For this review, take the finished solid that the model builds, in its own axes (mm). Face numbers are marked on the shaded views. A direction names the side the tool comes from. Coordinates: 2 decimals unless noted, no trailing zeros. Write each loop counter-clockwise with the first axis right and the second up, starting at its lowest first coordinate (ties: lowest second). Pieces come first, ordered by that corner, then holes.
```python
from build123d import *

# Parameters (mm, degrees)
SKETCH1_R                       = 6.35
BOSS_EXTRUDE1_DEPTH             = 25.4
F_21_0_159_DIAMETER_HOLE1_D     = 4.0386
F_21_0_159_DIAMETER_HOLE1_DEPTH = 9.0000074
F_21_0_159_DIAMETER_HOLE1_TIP   = 1.213317848
SKETCH5_W                       = 1.35255
SKETCH5_H                       = 6.35
SKETCH7_W                       = 12.7
SKETCH7_H                       = 3.96875


with BuildPart() as part:
    # Sketch1 → Boss-Extrude1 (new body)
    with BuildSketch(Plane(origin=(0, 0, 0), x_dir=(0, 0, -1), z_dir=(1, 0, 0))):
        Circle(SKETCH1_R)
    extrude(amount=BOSS_EXTRUDE1_DEPTH)

    # #21 (0.159) Diameter Hole1
    with Locations(Plane(origin=(25.4, 0, 0), x_dir=(0, 0, -1), z_dir=(1, 0, 0))):
        with Locations((0, 0)):
            Hole(F_21_0_159_DIAMETER_HOLE1_D / 2, depth=F_21_0_159_DIAMETER_HOLE1_DEPTH)
            with Locations((0, 0, -(F_21_0_159_DIAMETER_HOLE1_DEPTH + F_21_0_159_DIAMETER_HOLE1_TIP / 2))):  # 118° drill point
                Cone(0, F_21_0_159_DIAMETER_HOLE1_D / 2, F_21_0_159_DIAMETER_HOLE1_TIP, mode=Mode.SUBTRACT)

    # Sketch5 → #6-32 Tapped Hole1 (revolve, cut)
    with BuildSketch(Plane(origin=(20.32, 0, 0), x_dir=(0, 0, -1), z_dir=(1, 0, 0))):
        with Locations((0.676275, 3.175)):
            Rectangle(SKETCH5_W, SKETCH5_H)
    revolve(axis=Axis((20.32, -6.35, 0), (0, 1, 0)), mode=Mode.SUBTRACT)

    # Sketch7 → Cut-Revolve1 (revolve, cut)
    with BuildSketch(Plane(origin=(0, 0, 0), x_dir=(1, 0, 0), z_dir=(0, 1, 0))):
        with Locations((6.35, 4.365625)):
            Rectangle(SKETCH7_W, SKETCH7_H)
    revolve(axis=Axis((25.4, 0, 0), (-1, 0, 0)), mode=Mode.SUBTRACT)


solid = part.part
```
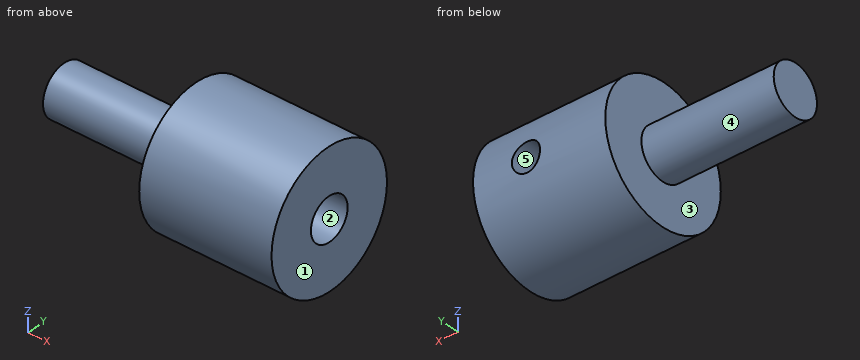
Q1. Draft analysis for pull direction Z (two halves, no side actions). For the marked faces 3, 4 and 5, state which applies: +Z half, -Z half, draft (parallel to the pull), parting line (faces both ways), or undercut.
Ans:
face 3: draft
face 4: parting line
face 5: undercut
Q2. Clearance check with flat-ended pins moving along their axes: pin 1 Ø2 at (x, z) = (17.5, 2.5) entering from +Y; pin 2 Ø4 at (x, z) = (3.5, 1.5) entering from +Y. State where each tip first meets the part, or that it passes through.
Ans:
pin 1: stops at y = 6.17
pin 2: stops at y = 2.38
Q3. For probe 1 along Z at (x, y) = (21.5, 0); probe 2 along X at (y, z) = (5.2, 0), list the stretches that pass through material, from the lowest coordinate up.
Ans:
probe 1: z = -6.35 to -2.02, 2.02 to 6.35
probe 2: x = 12.7 to 18.97, 21.67 to 25.4
Q4. Add section C-C (y = -5.25). State the section outline as (x, z) points, then the cut area to 3 significant figures.
Ans:
outline: (12.7, -3.57) - (25.4, -3.57) - (25.4, 3.57) - (12.7, 3.57) - close
area: 90.7 mm2
Q5. Add section B-B (z = 3.25). State the section outline as (x, y) points, then the cut area to 3 significant figures.
Ans:
outline: (12.7, -5.46) - (25.4, -5.46) - (25.4, 5.46) - (12.7, 5.46) - close
area: 139 mm2
Q6. Tool access review of the marked faces 1 and 2: name each direction out of +Z, -Z, +X, -X, +Y, -Y from which nothing blocks a thin tool from reaching the whole face with its end or side.
Ans:
face 1: +Z, -Z, +X, +Y, -Y
face 2: +X
Q7. Add section A-A (x = 22). State the section outline as (y, z) points, then the cut area to 3 significant figures.
Ans:
outline: circle Ø12.7 at (0, 0); hole circle Ø4.04 at (0, 0)
area: 114 mm2
